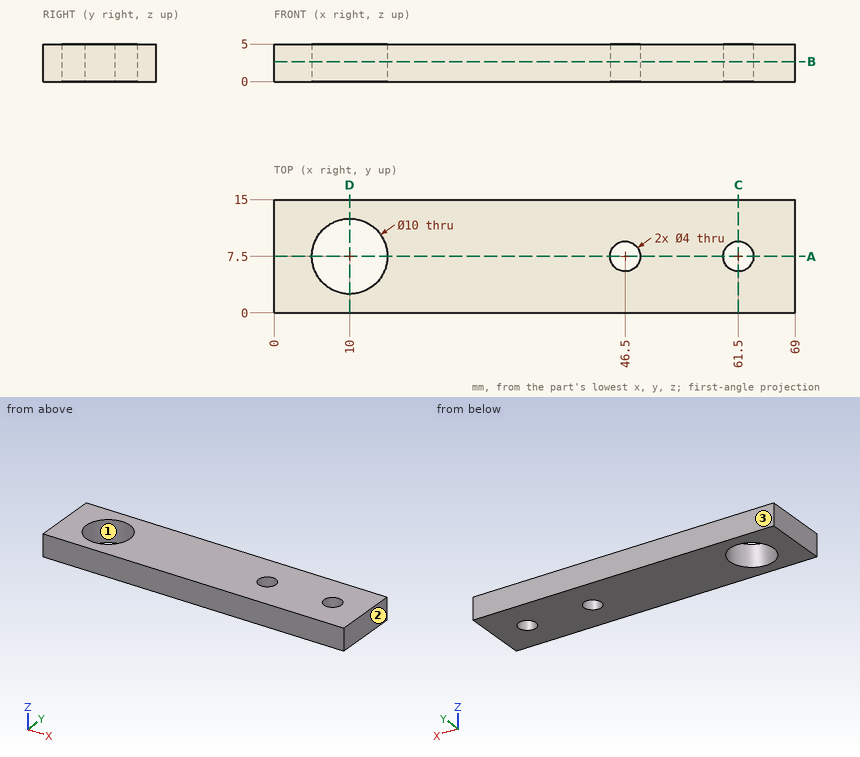
Here's the drawing with two shaded views (mm, measured from the low corner). I have some questions. Coordinates: 2 decimals unless noted, no trailing zeros. Write each loop counter-clockwise with the first axis right and the second up, starting at its lowest first coordinate (ties: lowest second). Pieces come first, ordered by that corner, then holes. Notation, with made-up numbers: (51, 75) -> (58, 75) arc R15 ccw to (58, 90) -> close; hole circle Ø6 at (44.5, 58). An arc over 180 degrees is marked (long way). Use a Markdown table: item, result. Add a question column.
(1) Please list where these lines run through material, in increasing order: line 1 (Y direction, x = 46.5, z = 3.05); line 2 (Y direction, x = 10, z = 1.35); line 3 (X direction, y = 8, z = 2.35).
(2) If we section it at B-B, the plane z = 2.65: Write out the boundary of the cut face in (x, y).
(3) If we section it at D-D, the plane x = 10: Write out the boundary of the cut face in (y, z), and give its area (3 significant figures).
(4) If we section it at A-A, the plane y = 7.5: Write out the boundary of the cut face in (x, z).
(5) We'd pull the mould along X, two halves only. Please class the marked faces 1, 2 and 3: +X half, -X half, draft (parallel to the pull), parting line (faces both ways), or undercut.
(6) If we section it at C-C, the plane x = 61.5: Write out the boundary of the cut face in (y, z).
Outcome:
| question | item | result |
|---|---|---|
| 1 | line 1 | y = 0 to 5.5, 9.5 to 15 |
| 1 | line 2 | y = 0 to 2.5, 12.5 to 15 |
| 1 | line 3 | x = 0 to 5.03, 14.97 to 44.56, 48.44 to 59.56, 63.44 to 69 |
| 2 | outline | (0, 0) -> (69, 0) -> (69, 15) -> (0, 15) -> close; hole circle Ø10 at (10, 7.5); hole circle Ø4 at (46.5, 7.5); hole circle Ø4 at (61.5, 7.5) |
| 3 | outline | (0, 0) -> (2.5, 0) -> (2.5, 5) -> (0, 5) -> close; (12.5, 0) -> (15, 0) -> (15, 5) -> (12.5, 5) -> close |
| 3 | area | 25.0 mm^2 |
| 4 | outline | (0, 0) -> (5, 0) -> (5, 5) -> (0, 5) -> close; (15, 0) -> (44.5, 0) -> (44.5, 5) -> (15, 5) -> close; (48.5, 0) -> (59.5, 0) -> (59.5, 5) -> (48.5, 5) -> close; (63.5, 0) -> (69, 0) -> (69, 5) -> (63.5, 5) -> close |
| 5 | face 1 | undercut |
| 5 | face 2 | +X half |
| 5 | face 3 | draft |
| 6 | outline | (0, 0) -> (5.5, 0) -> (5.5, 5) -> (0, 5) -> close; (9.5, 0) -> (15, 0) -> (15, 5) -> (9.5, 5) -> close |
